Could you check a few things on this model? Use its own coordinates, in mm. Face numbers are marked on the shaded views. A direction names the side the tool comes from. Give positions to 0.01 mm unless a question says otherwise; leave off trailing zeros. Write each loop counter-clockwise with the first axis right and the second up, starting at its lowest first coordinate (ties: lowest second). Pieces come first, ordered by that corner, then holes. Notation, with made-up numbers: (-11.75, 50.5) - (31.25, 50.5) arc R13 ccw to (31.25, 73.5) - close; hole circle Ø6 at (60.5, 2). An arc over 180 degrees is marked (long way). Answer in a Markdown table with one row per item.
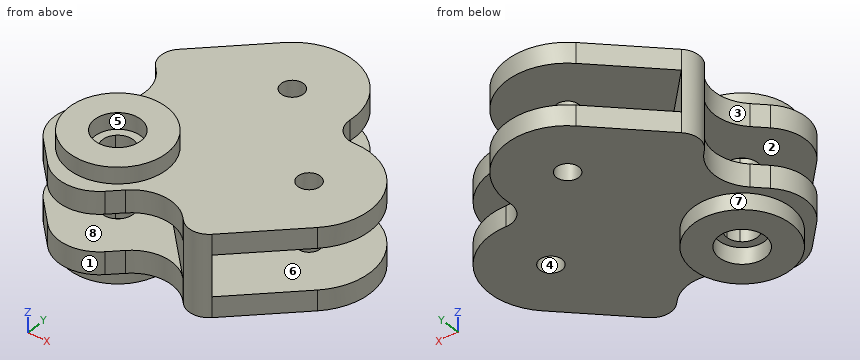
from build123d import *

# Parameters (mm, degrees)
SKETCH2_R               = 2.75
BOSS_EXTRUDE2_DEPTH     = 5
SKETCH3_R               = 2.75
BOSS_EXTRUDE3_DEPTH     = 5
SKETCH4_W               = 20
SKETCH4_H               = 60
BOSS_EXTRUDE4_DEPTH     = 5
FILLET1_R               = 5
SKETCH5_W               = 8
SKETCH5_H               = 10
BOSS_EXTRUDE5_DEPTH     = 20
FILLET3_START           = -16
FILLET3_DEPTH           = 22
CUT_EXTRUDE1_DEPTH      = 385.295668221
CUT_EXTRUDE1_DEPTH_BACK = 385.295668221
SKETCH8_R               = 9
SKETCH8_R_2             = 5.65
BOSS_EXTRUDE6_DEPTH     = 4
BOSS_EXTRUDE7_START     = 4
SKETCH9_R               = 9
SKETCH9_R_2             = 5.65
BOSS_EXTRUDE7_DEPTH     = 4
CUT_EXTRUDE2_DEPTH      = 2.5
CUT_EXTRUDE3_DEPTH      = 2.5
SKETCH12_W              = 5.5
SKETCH12_H              = 20
BOSS_EXTRUDE8_DEPTH     = 4
SKETCH13_W              = 5.5
SKETCH13_H              = 20
BOSS_EXTRUDE9_DEPTH     = 4
SKETCH14_W              = 5.5
SKETCH14_H              = 28
BOSS_EXTRUDE10_DEPTH    = 4
FILLET4_R               = 10
SKETCH16_R              = 12
SKETCH16_R_2            = 5.65
BOSS_EXTRUDE11_DEPTH    = 4
BOSS_EXTRUDE12_START    = 4
SKETCH17_R              = 12
SKETCH17_R_2            = 5.65
BOSS_EXTRUDE12_DEPTH    = 4


with BuildPart() as part:
    # Sketch2 → Boss-Extrude2 (new body)
    with BuildSketch(Plane.XY):
        with BuildLine():
            ThreePointArc((-79.393398282, 339.393398282), (-79.393398282, 360.606601718), (-100.606601718, 360.606601718))
            Line((-100.606601718, 360.606601718), (-115.031580054, 346.181623382))
            Line((-115.031580054, 346.181623382), (-72.605173183, 303.75521651))
            Line((-72.605173183, 303.75521651), (-58.180194847, 318.180194847))
            ThreePointArc((-58.180194847, 318.180194847), (-58.180194847, 339.393398282), (-79.393398282, 339.393398282))
        make_face()
        with Locations((-90, 350)):
            Circle(SKETCH2_R, mode=Mode.SUBTRACT)
        with Locations((-68.786796564, 328.786796564)):
            Circle(SKETCH2_R, mode=Mode.SUBTRACT)
    extrude(amount=BOSS_EXTRUDE2_DEPTH)



with BuildPart() as body_2:
    # Sketch3 → Boss-Extrude3 (new body)
    with BuildSketch(Plane(origin=(0, 0, -10), x_dir=(-1, 0, 0), z_dir=(0, 0, -1))):
        with BuildLine():
            Line((72.605173183, 303.75521651), (115.031580054, 346.181623382))
            Line((115.031580054, 346.181623382), (100.606601718, 360.606601718))
            ThreePointArc((100.606601718, 360.606601718), (79.393398282, 360.606601718), (79.393398282, 339.393398282))
            ThreePointArc((79.393398282, 339.393398282), (58.180194847, 339.393398282), (58.180194847, 318.180194847))
            Line((58.180194847, 318.180194847), (72.605173183, 303.75521651))
        make_face()
        with Locations(Location((90, 350, 0), (0, 0, 180))):
            Circle(SKETCH3_R, mode=Mode.SUBTRACT)
        with Locations(Location((68.786796564, 328.786796564, 0), (0, 0, 180))):
            Circle(SKETCH3_R, mode=Mode.SUBTRACT)
    extrude(amount=BOSS_EXTRUDE3_DEPTH)


with BuildPart() as part_1:
    add(part.part)

    add(body_2.part)  # Boss-Extrude4 merges body 2
    # Sketch4 → Boss-Extrude4 (add)
    with BuildSketch(Plane(origin=(115.575021664, 115.575021664, 0), x_dir=(0, 0, 1), z_dir=(-0.7071067811865471, -0.707106781186548, 0))):
        with Locations((-5, 296.126983722)):
            Rectangle(SKETCH4_W, SKETCH4_H)
    extrude(amount=BOSS_EXTRUDE4_DEPTH)

    # Fillet1
    fillet1_edges = [part_1.edges().sort_by_distance(p)[0] for p in [
        (-79.393398282, 339.393398282, 2.5),
        (-79.393398282, 339.393398282, -12.5),
    ]]
    fillet(fillet1_edges, radius=FILLET1_R)

    # Sketch5 → Boss-Extrude5 (add)
    with BuildSketch(Plane(origin=(112.039487758, 112.039487758, 0), x_dir=(0, 0, 1), z_dir=(-0.7071067811865477, -0.7071067811865475, 0))):
        with Locations((1, 301.126983722)):
            Rectangle(SKETCH5_W, SKETCH5_H)
        with Locations((-11, 301.126983722)):
            Rectangle(SKETCH5_W, SKETCH5_H)
        with Locations((-11, 291.126983722)):
            Rectangle(SKETCH5_W, SKETCH5_H)
        with Locations((1, 291.126983722)):
            Rectangle(SKETCH5_W, SKETCH5_H)
    extrude(amount=BOSS_EXTRUDE5_DEPTH)

    # Fillet3: read off the stored shape, not the designer's step
    # Fillet3 outline → Fillet3 (cut)
    with BuildSketch(Plane.XY.offset(FILLET3_START)):
        with BuildLine():
            Line((-118.56711396, 342.646089476), (-115.031580054, 339.11055557))
            ThreePointArc((-115.031580054, 339.11055557), (-116.496046148, 342.646089476), (-115.031580054, 346.181623382))
            Line((-115.031580054, 346.181623382), (-118.56711396, 342.646089476))
        make_face()
        with BuildLine():
            ThreePointArc((-72.605173183, 303.75521651), (-76.140707089, 302.290750416), (-79.676240995, 303.75521651))
            Line((-79.676240995, 303.75521651), (-76.140707089, 300.219682604))
            Line((-76.140707089, 300.219682604), (-72.605173183, 303.75521651))
        make_face()
    extrude(amount=FILLET3_DEPTH, mode=Mode.SUBTRACT)

    # Sketch7 → Cut-Extrude1 (cut, two sides: drawn at the far end of the back side and taken through both)
    with BuildSketch(Plane.XY.offset(5).offset(-CUT_EXTRUDE1_DEPTH_BACK)):
        with BuildLine():
            ThreePointArc((-100.674978336, 314.361818228), (-102.989915465, 317.826366475), (-107.076628766, 317.013468658))
            Line((-107.076628766, 317.013468658), (-101.773327907, 311.710167799))
            ThreePointArc((-101.773327907, 311.710167799), (-100.960430089, 312.926755357), (-100.674978336, 314.361818228))
        make_face()
        with BuildLine():
            Line((-101.773327907, 311.710167799), (-107.076628766, 317.013468658))
            ThreePointArc((-107.076628766, 317.013468658), (-107.076628766, 311.710167799), (-101.773327907, 311.710167799))
        make_face()
    extrude(amount=CUT_EXTRUDE1_DEPTH + CUT_EXTRUDE1_DEPTH_BACK, mode=Mode.SUBTRACT)

    # Sketch8 → Boss-Extrude6 (add)
    with BuildSketch(Plane(origin=(0, 0, -15), x_dir=(-1, 0, 0), z_dir=(0, 0, -1))):
        with Locations((104.424978336, 314.361818228)):
            Circle(SKETCH8_R)
        with Locations((104.424978336, 314.361818228)):
            Circle(SKETCH8_R_2, mode=Mode.SUBTRACT)
    extrude(amount=BOSS_EXTRUDE6_DEPTH)

    # Sketch9 → Boss-Extrude7 (add)
    with BuildSketch(Plane.XY.offset(5).offset(BOSS_EXTRUDE7_START)):
        with Locations(Location((-104.424978336, 314.361818228, 0), (0, 0, 180))):
            Circle(SKETCH9_R)
        with Locations(Location((-104.424978336, 314.361818228, 0), (0, 0, 180))):
            Circle(SKETCH9_R_2, mode=Mode.SUBTRACT)
    extrude(amount=-BOSS_EXTRUDE7_DEPTH)

    # Sketch10 → Cut-Extrude2 (cut)
    with BuildSketch(Plane.XY.offset(-7)):
        Polygon((-118.56711396, 314.361818228), (-104.424978336, 300.219682604), (-90.282842712, 314.361818228), (-104.424978336, 328.503953852), align=None)
    extrude(amount=-CUT_EXTRUDE2_DEPTH, mode=Mode.SUBTRACT)

    # Sketch11 → Cut-Extrude3 (cut)
    with BuildSketch(Plane(origin=(0, 0, -3), x_dir=(-1, 0, 0), z_dir=(0, 0, -1))):
        Polygon((90.282842712, 314.361818228), (104.424978336, 300.219682604), (118.56711396, 314.361818228), (104.424978336, 328.503953852), align=None)
    extrude(amount=-CUT_EXTRUDE3_DEPTH, mode=Mode.SUBTRACT)

    # Sketch12 → Boss-Extrude8 (add)
    with BuildSketch(Plane(origin=(-216.464466094, 216.464466094, 0), x_dir=(0, 0, 1), z_dir=(-0.7071067811865476, 0.7071067811865476, 0))):
        with Locations((-12.25, 148.447763109)):
            Rectangle(SKETCH12_W, SKETCH12_H)
        with Locations((2.25, 148.447763109)):
            Rectangle(SKETCH12_W, SKETCH12_H)
    extrude(amount=BOSS_EXTRUDE8_DEPTH)

    # Sketch13 → Boss-Extrude9 (add)
    with BuildSketch(Plane(origin=(-202.32233047, 202.32233047, 0), x_dir=(0, 0, -1), z_dir=(0.7071067811865476, -0.7071067811865476, 0))):
        with Locations((12.25, 148.447763109)):
            Rectangle(SKETCH13_W, SKETCH13_H)
        with Locations((-2.25, 148.447763109)):
            Rectangle(SKETCH13_W, SKETCH13_H)
    extrude(amount=BOSS_EXTRUDE9_DEPTH)

    # Sketch14 → Boss-Extrude10 (add)
    with BuildSketch(Plane(origin=(97.897352134, 97.897352134, 0), x_dir=(0, 0, 1), z_dir=(-0.7071067811865476, -0.7071067811865476, 0))):
        with Locations((2.25, 296.126983722)):
            Rectangle(SKETCH14_W, SKETCH14_H)
        with Locations((-12.25, 296.126983722)):
            Rectangle(SKETCH14_W, SKETCH14_H)
    extrude(amount=BOSS_EXTRUDE10_DEPTH)

    # Fillet4
    fillet4_edges = [part_1.edges().sort_by_distance(p)[0] for p in [
        (-107.253405461, 331.332380977, -12.25),
        (-107.253405461, 331.332380977, 2.25),
        (-87.454415588, 311.533391103, -12.25),
        (-87.454415588, 311.533391103, 2.25),
        (-104.424978336, 294.562828355, 2.25),
        (-124.223968209, 314.361818228, 2.25),
        (-124.223968209, 314.361818228, -12.25),
        (-104.424978336, 294.562828355, -12.25),
    ]]
    fillet(fillet4_edges, radius=FILLET4_R)

    # Sketch16 → Boss-Extrude11 (add)
    with BuildSketch(Plane(origin=(0, 0, -15), x_dir=(-1, 0, 0), z_dir=(0, 0, -1))):
        with Locations(Location((104.424978336, 314.361818228, 0), (0, 0, 180))):
            Circle(SKETCH16_R)
        with Locations((104.424978336, 314.361818228)):
            Circle(SKETCH16_R_2, mode=Mode.SUBTRACT)
    extrude(amount=BOSS_EXTRUDE11_DEPTH)

    # Sketch17 → Boss-Extrude12 (add)
    with BuildSketch(Plane.XY.offset(5).offset(BOSS_EXTRUDE12_START)):
        with Locations((-104.424978336, 314.361818228)):
            Circle(SKETCH17_R)
        with Locations(Location((-104.424978336, 314.361818228, 0), (0, 0, 180))):
            Circle(SKETCH17_R_2, mode=Mode.SUBTRACT)
    extrude(amount=-BOSS_EXTRUDE12_DEPTH)


solid = part_1.part
1) We'd pull the mould along X, two halves only. Please class the marked faces 1, 2, 3 and 4: +X half, -X half, draft (parallel to the pull), parting line (faces both ways), or undercut.
Check values:
| item | result |
|---|---|
| face 1 | parting line |
| face 2 | draft |
| face 3 | -X half |
| face 4 | undercut |
2) If I drill on line 1 (Z direction, x = -63, y = 313.5); line 2 (X direction, y = 314, z = 7); line 3 (Z direction, x = -107.5, y = 322), over which ranges is the centre line in solid material (lowest first)?
Check values:
| item | result |
|---|---|
| line 1 | z = -15 to -10, 0 to 5 |
| line 2 | x = -116.42 to -110.06, -98.79 to -92.43 |
| line 3 | z = -19 to -9.5, -0.5 to 9 |
3) Imagine slicing it at D-D (z = -1.75). List the corners of the cut face in (x, y) for me.
Check values:
| item | result |
|---|---|
| outline | (-115.03, 339.11) - (-79.68, 303.76) arc R5 ccw to (-72.61, 303.76) - (-115.03, 346.18) arc R5 ccw to start |
4) Imagine slicing it at B-B (x = -62.5). List the corners of the cut face in (y, z) for me, then the cut area to 3 significant figures.
Check values:
| item | result |
|---|---|
| outline | (313.86, -15) - (342.41, -15) - (342.41, -10) - (313.86, -10) - close; (313.86, 0) - (342.41, 0) - (342.41, 5) - (313.86, 5) - close |
| area | 285 mm2 |
5) Imagine slicing it at C-C (y = 350). List the corners of the cut face in (x, z) for me, then the cut area to 3 significant figures.
Check values:
| item | result |
|---|---|
| outline | (-111.21, -15) - (-92.75, -15) - (-92.75, -10) - (-111.21, -10) - close; (-111.21, 0) - (-92.75, 0) - (-92.75, 5) - (-111.21, 5) - close; (-87.25, -15) - (-75, -15) - (-75, -10) - (-87.25, -10) - close; (-87.25, 0) - (-75, 0) - (-75, 5) - (-87.25, 5) - close |
| area | 307 mm2 |
6) On a 3-axis mill with a long thin cutter (end or side, diameter ignored), from which of +Z, -Z, +X, -X, +Y, -Y can I reach the whole of each face in a straight line? I mean the marked faces 5, 6, 7 and 8. Say none if no direction works.
Check values:
| item | result |
|---|---|
| face 5 | +Z |
| face 6 | +X, +Y |
| face 7 | -Z |
| face 8 | -X, -Y |
7) Imagine slicing it at A-A (y = 361.5). List the corners of the cut face in (x, z) for me.
Check values:
| item | result |
|---|---|
| outline | (-99.63, -15) - (-80.37, -15) - (-80.37, -10) - (-99.63, -10) - close; (-99.63, 0) - (-80.37, 0) - (-80.37, 5) - (-99.63, 5) - close |
8) Will these pins go through, and if not, where does the flat tip stop? P1, Ø8, axis at y = 311.5, z = 4.5, coming from the +X side; P2, Ø9, axis at x = -90, y = 350, coming from the -Z side; P3, Ø4, axis at y = 328, z = -3.5, coming from the -X side; P4, Ø12.5, axis at x = -106, y = 312, coming from the -Z side.
Check values:
| item | result |
|---|---|
| P1 | stops at x = -60.86 |
| P2 | stops at z = -15 |
| P3 | stops at x = -105.92 |
| P4 | stops at z = -19 |
